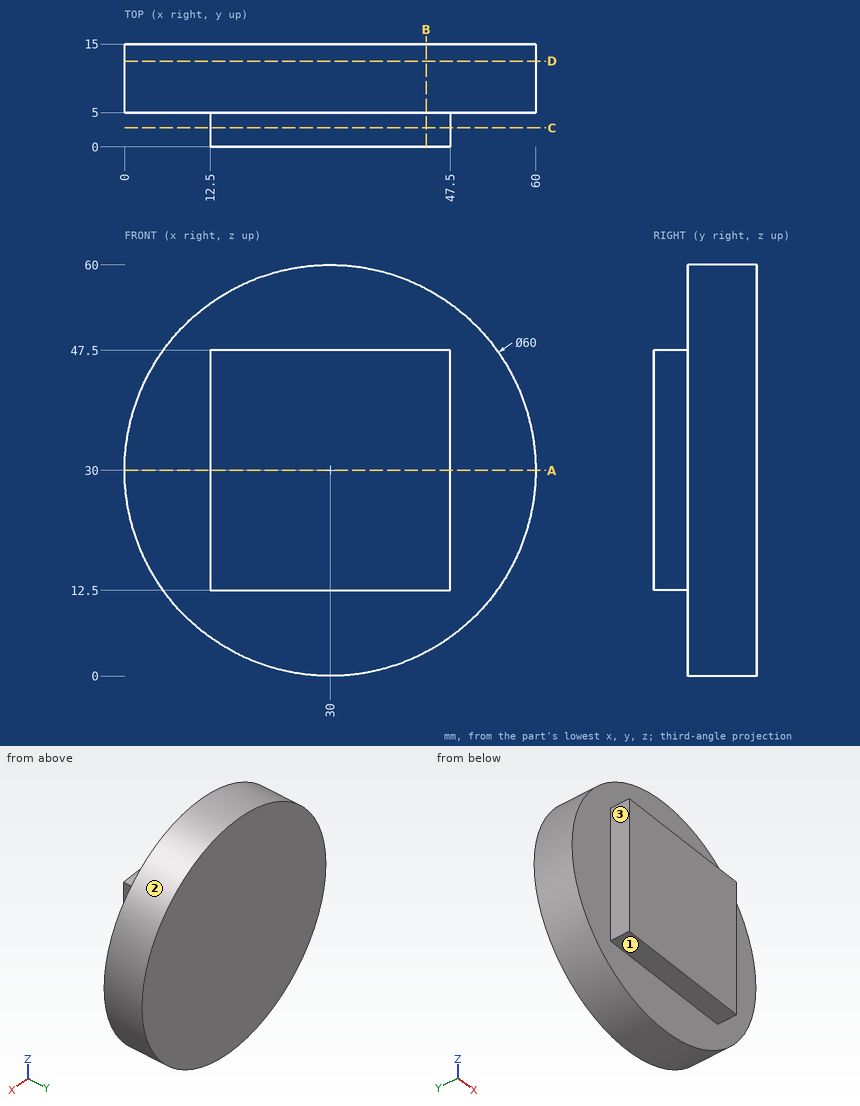
Part print with two shaded views. Sizes in mm from the minimum x, y, z corner. Coordinates: 2 decimals unless noted, no trailing zeros. Write each loop counter-clockwise with the first axis right and the second up, starting at its lowest first coordinate (ties: lowest second). Pieces come first, ordered by that corner, then holes.
(1) Cut at A-A on z = 30. List the corners of the cut face in (x, y), and give its area (3 significant figures).
(2) Cut at D-D on y = 12.5. List the corners of the cut face in (x, z).
(3) Drill centre lines: line 1 (Y direction, x = 48, z = 32); line 2 (Z direction, x = 42.5, y = 2). Where is each one in solid material? Low to high.
(4) Cut at B-B on x = 44. List the corners of the cut face in (y, z), and give its area (3 significant figures).
(5) Mould opens along X. For the marked faces 1, 2 and 3 say: pulls with the +X half, pulls with the -X half, needs draft (parallel to the pull), parting line crosses it, or undercut.
(6) Cut at C-C on y = 2.75. List the corners of the cut face in (x, z).
(7) Pin check, flat tips, straight feed: pin 1 Ø1 at (x, y) = (44.5, 6.5) entering from -Z; pin 2 Ø2.5 at (y, z) = (2.5, 24) entering from +X; pin 3 Ø1 at (x, z) = (7.5, 13.5) entering from -Y. Stop position of each tip, or through.
Working result:
1. outline: (0, 5) - (12.5, 5) - (12.5, 0) - (47.5, 0) - (47.5, 5) - (60, 5) - (60, 15) - (0, 15) - close
1. area: 775 mm2
2. outline: circle Ø60 at (30, 30)
3. line 1: y = 5 to 15
3. line 2: z = 12.5 to 47.5
4. outline: (0, 12.5) - (5, 12.5) - (5, 3.47) - (15, 3.47) - (15, 56.53) - (5, 56.53) - (5, 47.5) - (0, 47.5) - close
4. area: 706 mm2
5. face 1: needs draft
5. face 2: parting line crosses it
5. face 3: pulls with the -X half
6. outline: (12.5, 12.5) - (47.5, 12.5) - (47.5, 47.5) - (12.5, 47.5) - close
7. pin 1: stops at z = 3.47
7. pin 2: stops at x = 47.5
7. pin 3: stops at y = 5
